```python
from build123d import *

# Parameters (mm, degrees)
F0_W     = 100
F0_H     = 120
F0_W_2   = 10
F0_H_2   = 65
F0_R     = 3
F1_DEPTH = 8
F2_DEPTH = 80


with BuildPart() as f1:
    # F0 (on Top) → F1 (new body)
    with BuildSketch(Plane.XY):
        Rectangle(F0_W, F0_H)
        with Locations((0, -25.301723)):
            Rectangle(F0_W_2, F0_H_2, mode=Mode.SUBTRACT)
        with Locations((-28.999999, 13.00821)):
            Circle(F0_R, mode=Mode.SUBTRACT)
        with Locations((-29, 48.00821)):
            Circle(F0_R, mode=Mode.SUBTRACT)
        with Locations((29.000001, 13.00821)):
            Circle(F0_R, mode=Mode.SUBTRACT)
        with Locations((29, 48.00821)):
            Circle(F0_R, mode=Mode.SUBTRACT)
        with Locations((0, -25.301723)):
            Rectangle(F0_W_2, F0_H_2)
    extrude(amount=F1_DEPTH)

    # F0 (on Top) → F2 (join)
    with BuildSketch(Plane.XY):
        with Locations((0, -25.301723)):
            Rectangle(F0_W_2, F0_H_2)
    extrude(amount=F2_DEPTH)


solid = f1.part
```
Work out the finished part from the listing and answer in its coordinate system (mm). A direction names the side the tool comes from. Give positions to 0.01 mm unless a question says otherwise; leave off trailing zeros. Loops run counter-clockwise (first coordinate to the right, second up) from the corner with the lowest first, then second, coordinate; pieces in that order, holes last. Notation, with made-up numbers: (-39, -18) -> (-20, -18) arc R33 ccw to (-20, 12) -> close; hole circle Ø4 at (5, 27). An arc over 180 degrees is marked (long way). Write item = value, one per line. Start each with the question number.
(1) Find the intervals of material crossed by probe 1 along Y at (x, z) = (29, 5.5); probe 2 along Y at (x, z) = (1, 69.5); probe 3 along Y at (x, z) = (-27, 7), in increasing order. Write a range as from..to.
(2) Find section B-B on y = -41. Give the vertices of the cut face in (x, z), and give its area (3 significant figures).
(3) Find section A-A on x = -29. Give the vertices of the cut face in (y, z).
(4) Given pin 1 Ø8 at (x, z) = (-2.5, 61) entering from +Y; pin 2 Ø1 at (y, z) = (-26, 51) entering from +X; pin 3 Ø6 at (x, y) = (-10.5, -44.5) entering from +Z; pin 4 Ø9.5 at (x, y) = (-29, 48.01) entering from -Z, each flat-ended and moving along its own axis, determine where each tip first touches the part or whether it passes through.
(5) The mould has two halves that part along Y. Classify faces 1 (the cylindrical face through (26.789, 50.036, 3.944)), 2 (the flat face through (0, -25, 80)), 3 (the flat face through (-1, -60, 4)): +Y half, -Y half, draft (parallel to the pull), parting line (faces both ways), or undercut.
(6) Which of the six approach directions +Z, -Z, +X, -X, +Y, -Y give full straight-line access (tool end or side, diameter ignored) to faces 4 (the flat face through (0, 7.198, 43)), 5 (the cylindrical face through (31.77, 11.86, 3.94)), 6 (the flat face through (0, -57.802, 43)), 7 (the flat face through (5, -26, 43)), 8 (the flat face through (-5, -26, 43))?
(7) Find section D-D on x = 36. Give the vertices of the cut face in (y, z), and give its area (3 significant figures).
(8) Find section C-C on z = 71. Give the vertices of the cut face in (x, y).
From the geometry:
q1.probe_1 = -60..10.01, 16.01..45.01, 51.01..60
q1.probe_2 = -57.8..7.2
q1.probe_3 = -60..10.77, 15.24..45.77, 50.24..60
q2.outline = (-50, 0) -> (50, 0) -> (50, 8) -> (5, 8) -> (5, 80) -> (-5, 80) -> (-5, 8) -> (-50, 8) -> close
q2.area = 1,520 mm^2
q3.outline = (-60, 0) -> (10.01, 0) -> (10.01, 8) -> (-60, 8) -> close; (16.01, 0) -> (45.01, 0) -> (45.01, 8) -> (16.01, 8) -> close; (51.01, 0) -> (60, 0) -> (60, 8) -> (51.01, 8) -> close
q4.pin_1 = 7.2
q4.pin_2 = 5
q4.pin_3 = 8
q4.pin_4 = 0
q5.face_1 = undercut
q5.face_2 = draft
q5.face_3 = -Y half
q6.face_4 = +Z, +X, -X, +Y
q6.face_5 = +Z, -Z
q6.face_6 = +Z, +X, -X, -Y
q6.face_7 = +Z, +X, +Y, -Y
q6.face_8 = +Z, -X, +Y, -Y
q7.outline = (-60, 0) -> (60, 0) -> (60, 8) -> (-60, 8) -> close
q7.area = 960 mm^2
q8.outline = (-5, -57.8) -> (5, -57.8) -> (5, 7.2) -> (-5, 7.2) -> close
